from build123d import *

# Parameters (mm, degrees)
F0_W     = 50.8
F0_H     = 25.4
F1_DEPTH = 1778
F6_DEPTH = 50.8
F4_R     = 22.225
F7_DEPTH = 12.7
F8_R     = 19.05
F9_DEPTH = 50.8


with BuildPart() as f1:
    # F0 (on Front) → F1 (new body)
    with BuildSketch(Plane.XZ):
        with Locations((25.4, 12.7)):
            Rectangle(F0_W, F0_H)
    extrude(amount=F1_DEPTH)

    # F5 (on face) → F6 (join)
    with BuildSketch(Plane.YZ.offset(50.8)):
        with BuildLine():
            ThreePointArc((36.0393014908, 12.7), (20.46971854, 33.9050948807), (-4.424684912, 25.4))
            Line((-4.424684912, 25.4), (0, 25.4))
            Line((0, 25.4), (0, 0))
            Line((0, 0), (-4.424684912, 0))
            ThreePointArc((-4.424684912, 0), (20.46971854, -8.5050948807), (36.0393014908, 12.7))
        make_face()
        with BuildLine():
            Line((-1777.6152698337, 25.4), (-1773.575315088, 25.4))
            ThreePointArc((-1773.575315088, 25.4), (-1814.0393014908, 12.7), (-1773.575315088, 0))
            Line((-1773.575315088, 0), (-1777.6152698337, 0))
            ThreePointArc((-1777.6152698337, 0), (-1810.8643014908, 12.7), (-1777.6152698337, 25.4))
        make_face()
    extrude(amount=-F6_DEPTH)

    # F4 (on offset) → F7 (cut)
    with BuildSketch(Plane.YZ.offset(31.75)):
        with Locations((-1791.8143014908, 12.7)):
            Circle(F4_R)
        with Locations((13.8143014908, 12.7)):
            Circle(F4_R)
    extrude(amount=-F7_DEPTH, mode=Mode.SUBTRACT)

    # F8 (on face) → F9 (cut)
    with BuildSketch(Plane.YZ.offset(50.8)):
        with BuildLine():
            ThreePointArc((-1777.6152698337, 0), (-1774.0183180525, 5.9025391898), (-1772.7643014908, 12.7))
            ThreePointArc((-1772.7643014908, 12.7), (-1774.0183180525, 19.4974608102), (-1777.6152698337, 25.4))
            Line((-1777.6152698337, 25.4), (-1778, 25.4))
            Line((-1778, 25.4), (-1778, 0))
            Line((-1778, 0), (-1777.6152698337, 0))
        make_face()
        with Locations((13.8143014908, 12.7)):
            Circle(F8_R)
    extrude(amount=-F9_DEPTH, mode=Mode.SUBTRACT)


solid = f1.part
Input: part model. Units: mm. Frame: model coordinates. A direction names the side the tool comes from. Coordinates: 2 decimals unless noted, no trailing zeros. Loops run counter-clockwise (first coordinate to the right, second up) from the corner with the lowest first, then second, coordinate; pieces in that order, holes last.
Q1. Draft query along Y for faces 5 (the face through (9.658, -1814.025, 13.488)), 6 (the face through (50.8, -902, 13)). Return one class per face: +Y half, -Y half, draft (parallel to the pull), parting line (faces both ways), or undercut.
Q2. Cut plane A-A (x = 39.5). Output: boundary loops of the cut face in (y, z) (3 decimals).
Q3. Cut plane B-B (y = -959). Output: boundary loops of the cut face in (x, z), then the cut area to 3 significant figures.
Q4. Contact query for flat-ended pins moving along their axis: pin 1 (10 mm diameter, centred on x = 34.5, z = 30, fed in from -Y); pin 2 (10 mm diameter, centred on x = 5.5, y = -1609.5, fed in from +Z); pin 3 (3 mm diameter, centred on x = 23.5, z = 10, fed in from +Y). Output: stop coordinate, or through.
Q5. Set-up query: faces 1 (the face through (25, -877, 0)), 2 (the face through (25, -877, 25.4)), 3 (the face through (19.05, -1775, 23)), 4 (the face through (31.75, 32, 19)). Return all of +Z, -Z, +X, -X, +Y, -Y with unobstructed straight access to the full face (end or side cutting, diameter ignored); none if empty.
Q6. Material intervals for line 1 (Y direction, x = 42, z = 12); line 2 (Y direction, x = 15, z = 16); line 3 (Y direction, x = 33, z = 27), sorted ascending.
Working result:
1. face 5: undercut
1. face 6: draft
2. outline: (-1773.575, 0) - (-4.425, 0) arc R22.225 ccw (long way) to (-4.425, 25.4) - (-1773.575, 25.4) arc R22.225 ccw (long way) to start; hole circle Ø38.1 at (-1791.814, 12.7); hole circle Ø38.1 at (13.814, 12.7)
3. outline: (0, 0) - (50.8, 0) - (50.8, 25.4) - (0, 25.4) - close
3. area: 1,290 mm2
4. pin 1: stops at y = -1810.33
4. pin 2: stops at z = 25.4
4. pin 3: stops at y = -8.01
5. face 1: -Z, +X, -X
5. face 2: +Z, +X, -X
5. face 3: -Y
5. face 4: +Y
6. line 1: y = -1814.03 to -1810.85, -1772.78 to -5.22, 32.85 to 36.03
6. line 2: y = -1813.79 to -1810.58, -1773.05 to -4.95, 32.58 to 35.79
6. line 3: y = -1808.83 to -1804.4, -1779.23 to -1774.8, -3.2 to 1.23, 26.4 to 30.83
